from build123d import *

# Parameters (mm, degrees)
SKETCH4_R           = 39.6
SKETCH4_R_2         = 38.1
BOSS_EXTRUDE2_DEPTH = 599.44
SKETCH5_R           = 3.175
CUT_EXTRUDE1_DEPTH  = 603.050358027
CIRPATTERN1_COUNT   = 4
SKETCH6_R           = 3.175
CUT_EXTRUDE2_DEPTH  = 603.050358139
CIRPATTERN2_COUNT   = 4


with BuildPart() as part:
    # Sketch4 → Boss-Extrude2 (new body)
    with BuildSketch(Plane(origin=(0, 0, 0), x_dir=(1, 0, 0), z_dir=(0, 1, 0))):
        with Locations(Location((0, 0, 0), (0, 0, 270))):
            Circle(SKETCH4_R)
        with Locations(Location((0, 0, 0), (0, 0, 270))):
            Circle(SKETCH4_R_2, mode=Mode.SUBTRACT)
    extrude(amount=BOSS_EXTRUDE2_DEPTH)

    # Sketch5 → Cut-Extrude1 (cut, through all)
    with BuildSketch(Plane(origin=(0, 0, 0), x_dir=(0, 0, -1), z_dir=(1, 0, 0))):
        with Locations((0, 44.45)):
            Circle(SKETCH5_R)
    cut_extrude1 = extrude(amount=-CUT_EXTRUDE1_DEPTH, mode=Mode.SUBTRACT)

    # CirPattern1: Cut-Extrude1 ×4 about axis
    cirpattern1_axis = Axis((0, 599.44, 0), (0, -1, 0))
    for i in range(1, CIRPATTERN1_COUNT):
        add(cut_extrude1.rotate(cirpattern1_axis, i * 360 / CIRPATTERN1_COUNT), mode=Mode.SUBTRACT)

    # Sketch6 → Cut-Extrude2 (cut, through all)
    with BuildSketch(Plane(origin=(0, 0, 0), x_dir=(0, 0, -1), z_dir=(1, 0, 0))):
        with Locations(Location((0, 558.165, 0), (0, 0, 180))):
            Circle(SKETCH6_R)
    cut_extrude2 = extrude(amount=CUT_EXTRUDE2_DEPTH, mode=Mode.SUBTRACT)

    # CirPattern2: Cut-Extrude2 ×4 about axis
    cirpattern2_axis = Axis((0, 599.44, 0), (0, -1, 0))
    for i in range(1, CIRPATTERN2_COUNT):
        add(cut_extrude2.rotate(cirpattern2_axis, i * 360 / CIRPATTERN2_COUNT), mode=Mode.SUBTRACT)


solid = part.part
CAD build for the part. Positions are in the model's coordinates, mm. Round coordinates to 2 decimals unless told otherwise and drop trailing zeros. Order: outer loops, then holes, each group sorted by start corner. A loop starts at its lowest first (then second) coordinate and runs counter-clockwise, first axis right, second up. Notation, with made-up numbers: (55, 26.5) - (85, 26.5) arc R26 cw to (85, 46.5) - close; hole circle Ø10 at (14, 40.5). An arc over 180 degrees is marked (long way). Return JSON: item names as keys, results as strings.
(1) Pin check, flat tips, straight feed: pin 1 Ø8 at (y, z) = (148.5, 10) entering from -X; pin 2 Ø5 at (x, y) = (0, 558.165) entering from -Z; pin 3 Ø6 at (y, z) = (480.5, 22) entering from -X; pin 4 Ø12 at (y, z) = (443.5, 24.5) entering from -X. Stop position of each tip, or through.
Answer key:
{"pin 1": "stops at x = -39.14", "pin 2": "passes through", "pin 3": "stops at x = -34.74", "pin 4": "stops at x = -35.01"}
(2) Cut at C-C (y = 294.5). Give the cut face in (x, z), then the cut area to 3 significant figures.
Answer key:
{"outline": "circle Ø79.2 at (0, 0); hole circle Ø76.2 at (0, 0)", "area": "366 mm^2"}
(3) Pull direction X, two halves, no side cores. Call faces 1 (the face through (21, 0, -32)), 2 (the face through (11.895, 295.524, 37.771)), 3 (the face through (-23.183, 295.524, -30.235)): +X half, -X half, draft (parallel to the pull), parting line (faces both ways), or undercut.
Answer key:
{"face 1": "draft", "face 2": "parting line", "face 3": "undercut"}
(4) Cut at A-A (x = -13.5). Give the cut face in (y, z), then the cut area to 3 significant figures.
Answer key:
{"outline": "(0, -37.23) - (599.44, -37.23) - (599.44, -35.63) - (0, -35.63) - close; (0, 35.63) - (599.44, 35.63) - (599.44, 37.23) - (0, 37.23) - close", "area": "1,920 mm^2"}
(5) Cut at B-B (z = -13). Give the cut face in (x, y), then the cut area to 3 significant figures.
Answer key:
{"outline": "(-37.41, 0) - (-35.81, 0) - (-35.81, 599.44) - (-37.41, 599.44) - close; (35.81, 0) - (37.41, 0) - (37.41, 599.44) - (35.81, 599.44) - close", "area": "1,910 mm^2"}
(6) Wall check: probe 1 along Y at (x, z) = (39.25, 0) (3 decimals); probe 2 along Z at (x, y) = (0, 467); probe 3 along X at (y, z) = (250, -1). Give the ranges that are in metal, low to high. Write a range as from..to.
Answer key:
{"probe 1": "y = 0..41.275, 47.625..554.99, 561.34..599.44", "probe 2": "z = -39.6..-38.1, 38.1..39.6", "probe 3": "x = -39.59..-38.09, 38.09..39.59"}
